The model under review builds one solid part; all positions refer to its coordinate system, in mm. Give positions to 0.01 mm unless a question says otherwise; leave off trailing zeros. Loops run counter-clockwise (first coordinate to the right, second up) from the corner with the lowest first, then second, coordinate; pieces in that order, holes last. Notation, with made-up numbers: M 60,87.25 L 81,87.25 A28 ccw 81,116.25 Z; hole C 22,10 d2. An arc over 180 degrees is marked long. One line per item, written item: value. Start each with the question number.
Q1. To check wall thickness, follow line 1 along X through (y, z) = (-4.75, 72.27); line 2 along X through (y, z) = (-9.5, -1.5); line 3 along Z through (x, y) = (-33, -8.75). State the ranges of each line that lie inside material, in increasing order. Write a range as from..to.
Q2. We need section D-D on y = -6.25. Give the number of separate pieces and of enclosed holes in the cut face, plus the area to 3 significant figures.
Q3. For pin 1 (17 mm diameter, centred on x = -12.5, z = -72.73, fed in from +Y); pin 2 (23 mm diameter, centred on x = -7.5, z = 54.5, fed in from +Y); pin 3 (5 mm diameter, centred on x = 3, z = -101.5, fed in from -Y); pin 4 (6 mm diameter, centred on x = 24, y = -8.5, fed in from +Z), all flat-tipped, find the tip position at first contact; note any pin that passes through.
Q4. We need section A-A on x = 37.5. Write out the cut boundary in (y, z).
Q5. We need section B-B on z = 72.27. Write out the cut boundary in (x, y).
Q6. We need section C-C on x = -37.5. Write out the cut boundary in (y, z).
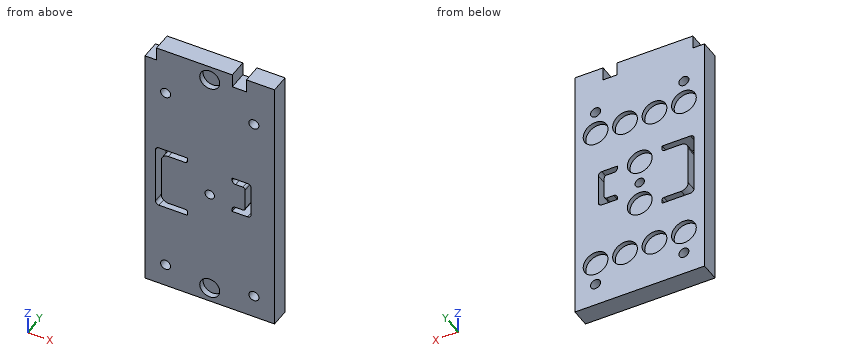
```python
from build123d import *

# Parameters (mm, degrees)
SKETCH1_W           = 110
SKETCH1_H           = 225
BOSS_EXTRUDE1_DEPTH = 16
CUT_EXTRUDE1_REACH  = 128.243
CUT_EXTRUDE2_REACH  = 128.243
SKETCH4_R           = 8.5
CUT_EXTRUDE3_DEPTH  = 5
SKETCH5_R           = 10.5
CUT_EXTRUDE4_DEPTH  = 4
CUT_EXTRUDE5_REACH  = 128.243
SKETCH6_W           = 12
SKETCH6_H           = 11.5
M10_TAPPED_HOLE1_D  = 8.5
CUT_EXTRUDE6_REACH  = 128.243
SKETCH10_R          = 4


with BuildPart() as part:
    # Sketch1 → Boss-Extrude1 (new body)
    with BuildSketch(Plane(origin=(0, 0, 0), x_dir=(1, 0, 0), z_dir=(0, 1, 0))):
        Rectangle(SKETCH1_W, SKETCH1_H)
    extrude(amount=-BOSS_EXTRUDE1_DEPTH)

    # Sketch2 → Cut-Extrude1 (cut, up to next)
    with BuildSketch(Plane(origin=(0, 0, 0), x_dir=(1, 0, 0), z_dir=(0, 1, 0)), mode=Mode.PRIVATE) as cut_extrude1_sk1:
        with BuildLine():
            Line((-19, 37.73), (-19, 34.23))
            ThreePointArc((-19, 34.23), (-19.439339828, 33.169339828), (-20.5, 32.73))
            Line((-20.5, 32.73), (-35.12, 32.73))
            ThreePointArc((-35.12, 32.73), (-39.362640687, 30.972640687), (-41.12, 26.73))
            Line((-41.12, 26.73), (-41.12, -6.27))
            ThreePointArc((-41.12, -6.27), (-39.362640687, -10.512640687), (-35.12, -12.27))
            Line((-35.12, -12.27), (-20.5, -12.27))
            ThreePointArc((-20.5, -12.27), (-19.439339828, -12.709339828), (-19, -13.77))
            Line((-19, -13.77), (-19, -17.27))
            Line((-19, -17.27), (-43.12, -17.27))
            ThreePointArc((-43.12, -17.27), (-45.241320344, -16.391320344), (-46.12, -14.27))
            Line((-46.12, -14.27), (-46.12, 34.73))
            ThreePointArc((-46.12, 34.73), (-45.241320344, 36.851320344), (-43.12, 37.73))
            Line((-43.12, 37.73), (-19, 37.73))
        make_face()
    cut_extrude1_tool1 = extrude(cut_extrude1_sk1.sketch, amount=-CUT_EXTRUDE1_REACH, mode=Mode.PRIVATE) & part.part
    add(cut_extrude1_tool1.solids().sort_by_distance((-44.807702, 0, 15.957702))[0], mode=Mode.SUBTRACT)

    # Sketch3 → Cut-Extrude2 (cut, up to next)
    with BuildSketch(Plane(origin=(0, 0, 0), x_dir=(1, 0, 0), z_dir=(0, 1, 0)), mode=Mode.PRIVATE) as cut_extrude2_sk1:
        with BuildLine():
            Line((19, 18.73), (32.13, 18.73))
            ThreePointArc((32.13, 18.73), (34.251320344, 17.851320344), (35.13, 15.73))
            Line((35.13, 15.73), (35.13, -10.27))
            ThreePointArc((35.13, -10.27), (34.251320344, -12.391320344), (32.13, -13.27))
            Line((32.13, -13.27), (19, -13.27))
            Line((19, -13.27), (19, -11.27))
            ThreePointArc((19, -11.27), (19.878679656, -9.148679656), (22, -8.27))
            Line((22, -8.27), (28.13, -8.27))
            ThreePointArc((28.13, -8.27), (29.544213562, -7.684213562), (30.13, -6.27))
            Line((30.13, -6.27), (30.13, 11.73))
            ThreePointArc((30.13, 11.73), (29.544213562, 13.144213562), (28.13, 13.73))
            Line((28.13, 13.73), (22, 13.73))
            ThreePointArc((22, 13.73), (19.878679656, 14.608679656), (19, 16.73))
            Line((19, 16.73), (19, 18.73))
        make_face()
    cut_extrude2_tool1 = extrude(cut_extrude2_sk1.sketch, amount=-CUT_EXTRUDE2_REACH, mode=Mode.PRIVATE) & part.part
    add(cut_extrude2_tool1.solids().sort_by_distance((29.797608, 0, -13.397608))[0], mode=Mode.SUBTRACT)

    # Sketch4 → Cut-Extrude3 (cut)
    with BuildSketch(Plane.XZ.offset(16)):
        with Locations(Location((0, 100, 0), (0, 0, 270))):
            Circle(SKETCH4_R)
        with Locations(Location((0, -100, 0), (0, 0, 270))):
            Circle(SKETCH4_R)
    extrude(amount=-CUT_EXTRUDE3_DEPTH, mode=Mode.SUBTRACT)

    # Sketch5 → Cut-Extrude4 (cut)
    with BuildSketch(Plane(origin=(0, 0, 0), x_dir=(1, 0, 0), z_dir=(0, 1, 0))):
        with Locations(Location((-37.5, 72.73, 0), (0, 0, 270))):
            Circle(SKETCH5_R)
        with Locations(Location((-12.5, 72.73, 0), (0, 0, 270))):
            Circle(SKETCH5_R)
        with Locations(Location((12.5, 72.73, 0), (0, 0, 270))):
            Circle(SKETCH5_R)
        with Locations(Location((37.5, 72.73, 0), (0, 0, 270))):
            Circle(SKETCH5_R)
        with Locations(Location((37.5, -52.27, 0), (0, 0, 90))):
            Circle(SKETCH5_R)
        with Locations(Location((12.5, -52.27, 0), (0, 0, 90))):
            Circle(SKETCH5_R)
        with Locations(Location((-12.5, -52.27, 0), (0, 0, 90))):
            Circle(SKETCH5_R)
        with Locations(Location((-37.5, -52.27, 0), (0, 0, 90))):
            Circle(SKETCH5_R)
        with Locations(Location((0, 30.23, 0), (0, 0, 270))):
            Circle(SKETCH5_R)
        with Locations(Location((0, -9.77, 0), (0, 0, 270))):
            Circle(SKETCH5_R)
    extrude(amount=-CUT_EXTRUDE4_DEPTH, mode=Mode.SUBTRACT)

    # Sketch6 → Cut-Extrude5 (cut, up to next)
    with BuildSketch(Plane(origin=(0, 0, 0), x_dir=(1, 0, 0), z_dir=(0, 1, 0)), mode=Mode.PRIVATE) as cut_extrude5_sk1:
        with Locations((25.13, -106.75)):
            Rectangle(SKETCH6_W, SKETCH6_H)
    cut_extrude5_tool1 = extrude(cut_extrude5_sk1.sketch, amount=-CUT_EXTRUDE5_REACH, mode=Mode.PRIVATE) & part.part
    # Sketch6 → Cut-Extrude5 (cut, up to next)
    with BuildSketch(Plane(origin=(0, 0, 0), x_dir=(1, 0, 0), z_dir=(0, 1, 0)), mode=Mode.PRIVATE) as cut_extrude5_sk2:
        with Locations((-51.12, -106.75)):
            Rectangle(SKETCH6_W, SKETCH6_H)
    cut_extrude5_tool2 = extrude(cut_extrude5_sk2.sketch, amount=-CUT_EXTRUDE5_REACH, mode=Mode.PRIVATE) & part.part
    add(cut_extrude5_tool1.solids().sort_by_distance((25.13, 0, 106.75))[0], mode=Mode.SUBTRACT)
    add(cut_extrude5_tool2.solids().sort_by_distance((-51.12, 0, 106.75))[0], mode=Mode.SUBTRACT)

    # M10 Tapped Hole1 (through all)
    with Locations(Plane(origin=(0, 0, 0), x_dir=(1, 0, 0), z_dir=(0, 1, 0))):
        with Locations((-37.5, -72.27), (37.5, -72.27), (37.5, 92.73), (-37.5, 92.73)):
            Hole(M10_TAPPED_HOLE1_D / 2)

    # Sketch10 → Cut-Extrude6 (cut, up to next)
    with BuildSketch(Plane(origin=(0, 0, 0), x_dir=(1, 0, 0), z_dir=(0, 1, 0)), mode=Mode.PRIVATE) as cut_extrude6_sk1:
        with Locations(Location((0, 10.23, 0), (0, 0, 270))):
            Circle(SKETCH10_R)
    cut_extrude6_tool1 = extrude(cut_extrude6_sk1.sketch, amount=-CUT_EXTRUDE6_REACH, mode=Mode.PRIVATE) & part.part
    add(cut_extrude6_tool1.solids().sort_by_distance((0, 0, -10.23))[0], mode=Mode.SUBTRACT)


solid = part.part
```
Solved:
1. line 1: -55..-41.75, -33.25..33.25, 41.75..55
1. line 2: -55..-46.12, -41.12..30.13, 35.13..55
1. line 3: -112.5..-37.73, -32.73..12.27, 17.27..112.5
2. separate pieces: 1
2. enclosed holes: 7
2. area: 23,400 mm2
3. pin 1: y = -4
3. pin 2: y = 0
3. pin 3: y = -11
3. pin 4: z = 101
4. outline: M -16,-112.5 L 0,-112.5 L 0,-96.98 L -16,-96.98 Z; M -16,-88.48 L 0,-88.48 L 0,-83.23 L -4,-83.23 L -4,-62.23 L 0,-62.23 L 0,41.77 L -4,41.77 L -4,62.77 L 0,62.77 L 0,68.02 L -16,68.02 Z; M -16,76.52 L 0,76.52 L 0,112.5 L -16,112.5 Z
5. outline: M -55,-16 L -41.75,-16 L -41.75,0 L -55,0 Z; M -33.25,-16 L 33.25,-16 L 33.25,0 L -33.25,0 Z; M 41.75,-16 L 55,-16 L 55,0 L 41.75,0 Z
6. outline: M -16,-112.5 L 0,-112.5 L 0,-96.98 L -16,-96.98 Z; M -16,-88.48 L 0,-88.48 L 0,-83.23 L -4,-83.23 L -4,-62.23 L 0,-62.23 L 0,-37.73 L -16,-37.73 Z; M -16,-32.24 L 0,-32.24 L 0,11.78 L -16,11.78 Z; M -16,17.27 L 0,17.27 L 0,41.77 L -4,41.77 L -4,62.77 L 0,62.77 L 0,68.02 L -16,68.02 Z; M -16,76.52 L 0,76.52 L 0,112.5 L -16,112.5 Z
